Design review of the part built by this model. Coordinates are the model's own, in mm. A direction names the side the tool comes from. Give positions to 0.01 mm unless a question says otherwise; leave off trailing zeros. Write each loop counter-clockwise with the first axis right and the second up, starting at its lowest first coordinate (ties: lowest second). Pieces come first, ordered by that corner, then holes. Notation, with made-up numbers: M 60.5,48 L 112.5,48 A13 cw 112.5,54 Z; hole C 67,9.25 d6. An arc over 180 degrees is marked long. Write each question's results on one line, items separated by ' | '. Start each with the question number.
from build123d import *

# Parameters (mm, degrees)
SKETCH1_R               = 6.9
SKETCH1_R_2             = 5.4
BOSS_EXTRUDE1_DEPTH     = 7.3
SKETCH2_R               = 6.9
BOSS_EXTRUDE2_DEPTH     = 2.2
FILLET1_R               = 2
SKETCH6_W               = 1.1
SKETCH6_H               = 1
SKETCH4_W               = 5
SKETCH4_H               = 4.8
CUT_EXTRUDE1_DEPTH      = 14.618737093
CUT_EXTRUDE2_DEPTH      = 14.618737093
CUT_EXTRUDE2_DEPTH_BACK = 14.618737093
SKETCH5_W               = 1.5
SKETCH5_H               = 4.5
SKETCH3_R               = 3
BOSS_EXTRUDE3_DEPTH     = 3


with BuildPart() as part:
    # Sketch1 → Boss-Extrude1 (new body)
    with BuildSketch(Plane(origin=(0, 0, 0), x_dir=(1, 0, 0), z_dir=(0, 1, 0))):
        with Locations(Location((0, 0, 0), (0, 0, 270))):
            Circle(SKETCH1_R)
        with Locations(Location((0, 0, 0), (0, 0, 270))):
            Circle(SKETCH1_R_2, mode=Mode.SUBTRACT)
    extrude(amount=BOSS_EXTRUDE1_DEPTH)

    # Sketch2 → Boss-Extrude2 (add)
    with BuildSketch(Plane(origin=(0, 7.3, 0), x_dir=(1, 0, 0), z_dir=(0, 1, 0))):
        with Locations(Location((0, 0, 0), (0, 0, 270))):
            Circle(SKETCH2_R)
    extrude(amount=BOSS_EXTRUDE2_DEPTH)

    # Fillet1
    fillet1_edges = [part.edges().sort_by_distance(p)[0] for p in [
        (0, 9.5, -6.9),
    ]]
    fillet(fillet1_edges, radius=FILLET1_R)

    # Sketch6 → Revolve3 (revolve)
    with BuildSketch(Plane.XY, mode=Mode.PRIVATE) as revolve3_sk:
        with Locations((4.95, 4.3)):
            Rectangle(SKETCH6_W, SKETCH6_H)
    revolve(revolve3_sk.sketch.rotate(Axis((0, 9.975, 0), (0, -1, 0)), 90), axis=Axis((0, 9.975, 0), (0, -1, 0)))

    # Sketch4 → Cut-Extrude1 (cut, through all)
    with BuildSketch(Plane.XY):
        with Locations((0, 2.4)):
            Rectangle(SKETCH4_W, SKETCH4_H)
    extrude(amount=CUT_EXTRUDE1_DEPTH, mode=Mode.SUBTRACT)

    # Sketch5 → Cut-Extrude2 (cut, two sides: drawn at the far end of the back side and taken through both)
    with BuildSketch(Plane(origin=(0, 0, 0), x_dir=(0, 0, -1), z_dir=(1, 0, 0)).offset(-CUT_EXTRUDE2_DEPTH_BACK)):
        with Locations((0, 2.25)):
            Rectangle(SKETCH5_W, SKETCH5_H)
    extrude(amount=CUT_EXTRUDE2_DEPTH + CUT_EXTRUDE2_DEPTH_BACK, mode=Mode.SUBTRACT)

    # Sketch3 → Boss-Extrude3 (add)
    with BuildSketch(Plane.XZ.offset(-7.3)):
        with Locations(Location((0, 0, 0), (0, 0, 90))):
            Circle(SKETCH3_R)
    extrude(amount=BOSS_EXTRUDE3_DEPTH)


solid = part.part
Q1. Wall thickness on line 1 along X through (y, z) = (5.5, 0); line 2 along Y through (x, z) = (-3.75, 2.5); line 3 along Y through (x, z) = (1, 2): over which ranges is each line inside the solid? List them lowest first. Write a range as from..to.
Q2. We need section A-A on y = 2.5. Write out the cut boundary in (x, z), and give its area (3 significant figures).
Q3. For pin 1 Ø1.3 at (x, y) = (6, 3) entering from +Z; pin 2 Ø1.5 at (y, z) = (7.5, 3.5) entering from -X; pin 3 Ø3 at (x, y) = (-6, 1) entering from -Z, all flat-tipped, find the tip position at first contact; note any pin that passes through.
Q4. We need section C-C on y = 7. Write out the cut boundary in (x, z).
Q5. The part is to be moulded in two halves that separate along Z. For faces 1 (the flat face through (0, 0, -6)), 2 (the flat face through (-6, 2, 0.75)), 3 (the flat face through (6, 4.5, 0)), 4 (the cylindrical face through (0.303, 3.698, -6.893)), say which applies: pulls with the +Z half, pulls with the -Z half, needs draft (parallel to the pull), parting line crosses it, or undercut.
Q6. We need section B-B on z = 0. Write out the cut boundary in (x, y), and give its area (3 significant figures).
Q7. We need section D-D on x = 0. Write out the cut boundary in (y, z), and give its area (3 significant figures).
Q8. For faces 5 (the flat face through (0, 4.8, 6)), 6 (the flat face through (-2.3, 7.3, 2.3)), 7 (the flat face through (0, 3.8, -5)), list the 3-axis set-ups (+Z, -Z, +X, -X, +Y, -Y) from which the entire face can be reached by the end or side of a thin tool; tool diameter is ignored.
Answer sheet:
1) line 1: -6.9..-5.4, -3..3, 5.4..6.9 | line 2: 3.8..4.8, 7.3..9.5 | line 3: 4.3..9.5
2) outline: M -6.86,-0.75 A6.9 ccw 6.86,-0.75 L 5.35,-0.75 A5.4 cw -5.35,-0.75 Z; M -6.86,0.75 L -5.35,0.75 A5.4 cw -2.5,4.79 L -2.5,6.43 A6.9 ccw Z; M 2.5,4.79 A5.4 cw 5.35,0.75 L 6.86,0.75 A6.9 ccw 2.5,6.43 Z | area: 45.7 mm^2
3) pin 1: z = 4.36 | pin 2: x = -6.33 | pin 3: z = -5.23
4) outline: C 0,0 d13.8; C 0,0 d6; hole C 0,0 d10.8
5) face 1: needs draft | face 2: undercut | face 3: undercut | face 4: parting line crosses it
6) outline: M -6.9,4.5 L -4.4,4.5 L -4.4,4.8 L -5.4,4.8 L -5.4,7.3 L -3,7.3 L -3,4.3 L 3,4.3 L 3,7.3 L 5.4,7.3 L 5.4,4.8 L 4.4,4.8 L 4.4,4.5 L 6.9,4.5 L 6.9,7.5 A2 ccw 4.9,9.5 L -4.9,9.5 A2 ccw -6.9,7.5 Z | area: 55.6 mm^2
7) outline: M 0,-6.9 L 7.5,-6.9 A2 ccw 9.5,-4.9 L 9.5,4.9 A2 ccw 7.5,6.9 L 4.8,6.9 L 4.8,5.4 L 7.3,5.4 L 7.3,3 L 4.3,3 L 4.3,-3 L 7.3,-3 L 7.3,-5.4 L 4.8,-5.4 L 4.8,-4.4 L 3.8,-4.4 L 3.8,-5.4 L 0,-5.4 Z | area: 62.3 mm^2
8) face 5: +Z, -Y | face 6: none | face 7: -Y
